```python
from build123d import *

# Parameters (mm, degrees)
SKETCH1_R           = 25
BOSS_EXTRUDE1_DEPTH = 15
CUT_EXTRUDE1_START  = -10
SKETCH2_R           = 5
CUT_EXTRUDE1_DEPTH  = 60
SKETCH8_R           = 20
BOSS_EXTRUDE4_DEPTH = 5
SKETCH3_R           = 1.5
CUT_EXTRUDE2_DEPTH  = 20
CIRPATTERN2_COUNT   = 4
SKETCH4_R           = 12.5
BOSS_EXTRUDE2_DEPTH = 30
CUT_EXTRUDE4_START  = -5
SKETCH7_R           = 1.5
CUT_EXTRUDE4_DEPTH  = 15
FILLET3_R           = 2


with BuildPart() as part:
    # Sketch1 → Boss-Extrude1 (new body)
    with BuildSketch(Plane.XY):
        Circle(SKETCH1_R)
    extrude(amount=BOSS_EXTRUDE1_DEPTH)

    # Sketch2 → Cut-Extrude1 (cut)
    with BuildSketch(Plane(origin=(0, 0, 0), x_dir=(1, 0, 0), z_dir=(0, 1, 0)).offset(CUT_EXTRUDE1_START)):
        with Locations(Location((0, -7, 0), (0, 0, 270))):
            Circle(SKETCH2_R)
    cut_extrude1 = extrude(amount=-CUT_EXTRUDE1_DEPTH, mode=Mode.SUBTRACT)

    # Sketch8 → Boss-Extrude4 (add)
    with BuildSketch(Plane(origin=(0, 0, 0), x_dir=(-1, 0, 0), z_dir=(0, 0, -1))):
        Circle(SKETCH8_R)
    extrude(amount=BOSS_EXTRUDE4_DEPTH)

    # Sketch3 → Cut-Extrude2 (cut)
    with BuildSketch(Plane.XY.offset(15)):
        with Locations((0, -17.5)):
            Circle(SKETCH3_R)
    cut_extrude2 = extrude(amount=-CUT_EXTRUDE2_DEPTH, mode=Mode.SUBTRACT)

    # CirPattern2: Cut-Extrude1, Cut-Extrude2 ×4 about axis
    cirpattern2_axis = Axis((0, 0, 0), (0, 0, 1))
    add([cut_extrude1.rotate(cirpattern2_axis, i * 360 / CIRPATTERN2_COUNT) for i in range(1, CIRPATTERN2_COUNT)], mode=Mode.SUBTRACT)
    add([cut_extrude2.rotate(cirpattern2_axis, i * 360 / CIRPATTERN2_COUNT) for i in range(1, CIRPATTERN2_COUNT)], mode=Mode.SUBTRACT)

    # Sketch4 → Boss-Extrude2 (add)
    with BuildSketch(Plane(origin=(0, 0, 0), x_dir=(-1, 0, 0), z_dir=(0, 0, -1))):
        Circle(SKETCH4_R)
    extrude(amount=BOSS_EXTRUDE2_DEPTH)

    # Sketch7 → Cut-Extrude4 (cut)
    with BuildSketch(Plane(origin=(0, 0, 0), x_dir=(0, 0, -1), z_dir=(1, 0, 0)).offset(CUT_EXTRUDE4_START)):
        with Locations((27, 0)):
            Circle(SKETCH7_R)
    extrude(amount=-CUT_EXTRUDE4_DEPTH, mode=Mode.SUBTRACT)

    # Fillet3
    fillet3_edges = [part.edges().sort_by_distance(p)[0] for p in [
        (12.5, 0, -5),
    ]]
    fillet(fillet3_edges, radius=FILLET3_R)


solid = part.part
```
For this review, take the finished solid that the model builds, in its own axes (mm). A direction names the side the tool comes from. Coordinates: 2 decimals unless noted, no trailing zeros. Write each loop counter-clockwise with the first axis right and the second up, starting at its lowest first coordinate (ties: lowest second). Pieces come first, ordered by that corner, then holes.
(1) Wall thickness on probe 1 along Z at (x, y) = (20.5, 0); probe 2 along Z at (x, y) = (-6.75, 0); probe 3 along Z at (x, y) = (21, 13): over which ranges is each line inside the solid? List them lowest first.
(2) Tool access review of faces 4 (the face through (-8.7, 0.07, -25.5)), 5 (the face through (17.395, -1.915, 11.619)), 6 (the face through (0, 10, 7)): name each direction out of +Z, -Z, +X, -X, +Y, -Y from which nothing blocks a thin tool from reaching the whole face with its end or side.
(3) Add section D-D on z = 3. Give the boundary of the cut face in (x, y), then the cut area to 3 significant figures.
(4) The part is to be moulded in two halves that separate along Y. For faces 1 (the face through (0, -10, 7)), 2 (the face through (1.43, -17.05, 13.41)), 3 (the face through (0, 0, 15)), say which applies: +Y half, -Y half, draft (parallel to the pull), parting line (faces both ways), or undercut.
(5) For pin 1 Ø3 at (y, z) = (-1.5, 5.5) entering from -X; pin 2 Ø3 at (x, z) = (2, 5) entering from -Y; pin 3 Ø3 at (y, z) = (3.5, 10) entering from +X, all flat-tipped, find the tip position at first contact; note any pin that passes through.
(6) Add section C-C on x = 0. Count the separate pieces of the cut face and the enclosed holes in it, then the cut area to 3 significant figures.
(7) Add section A-A on x = -17.5. Give the boundary of the cut face in (y, z), then the cut area to 3 significant figures.
Answer sheet:
1. probe 1: z = 0 to 2, 12 to 15
1. probe 2: z = -30 to -28.5, -25.5 to 15
1. probe 3: z = 0 to 15
2. face 4: -X
2. face 5: +X
2. face 6: +Y
3. outline: (-24.82, -3) arc R25 ccw to (-3, -24.82) - (-3, -10) - (3, -10) - (3, -24.82) arc R25 ccw to (24.82, -3) - (10, -3) - (10, 3) - (24.82, 3) arc R25 ccw to (3, 24.82) - (3, 10) - (-3, 10) - (-3, 24.82) arc R25 ccw to (-24.82, 3) - (-10, 3) - (-10, -3) - close
3. area: 1,600 mm2
4. face 1: -Y half
4. face 2: undercut
4. face 3: draft
5. pin 1: stops at x = -10
5. pin 2: stops at y = -10
5. pin 3: stops at x = 24.86
6. separate pieces: 5
6. enclosed holes: 0
6. area: 1,220 mm2
7. outline: (-17.85, 0) - (-9.68, 0) - (-9.68, -5) - (-1.5, -5) - (-1.5, 2.23) arc R5 cw to (-1.5, 11.77) - (-1.5, 15) - (-17.85, 15) - close; (1.5, -5) - (9.68, -5) - (9.68, 0) - (17.85, 0) - (17.85, 15) - (1.5, 15) - (1.5, 11.77) arc R5 cw to (1.5, 2.23) - close
7. area: 523 mm2
